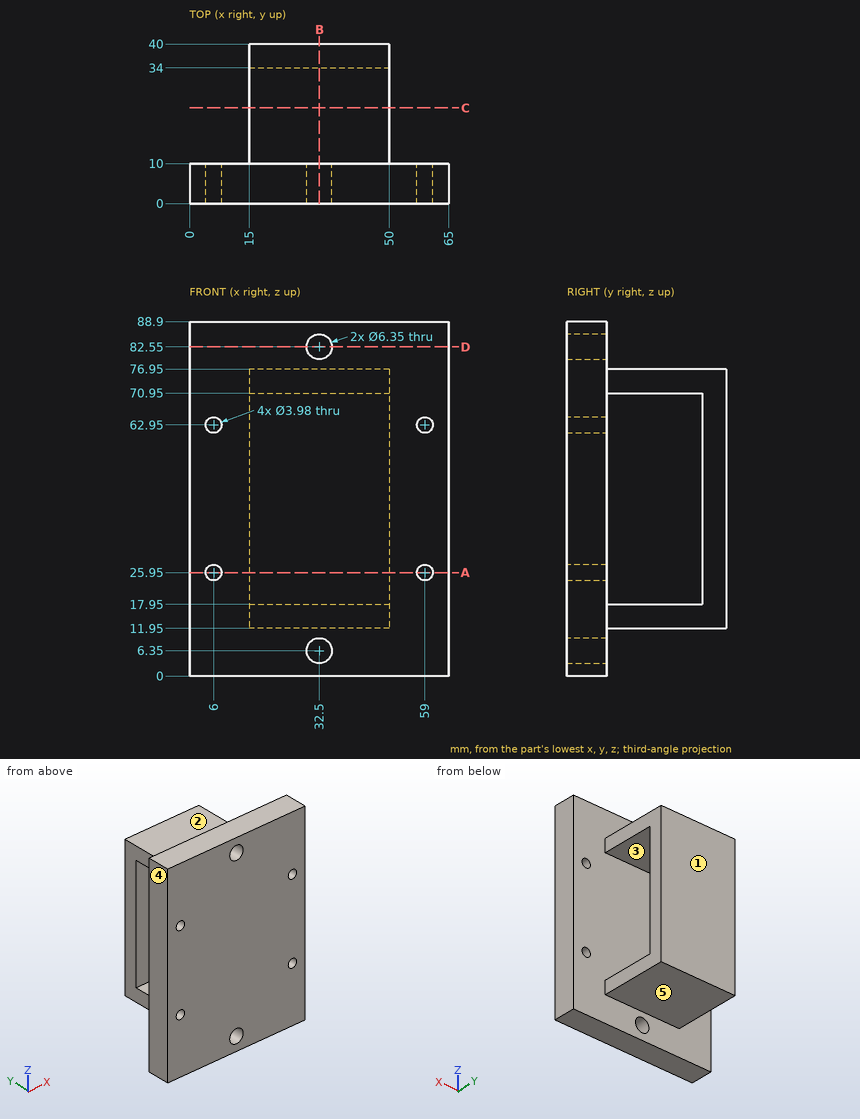
Answer from the drawing. Dimensions are ordinates in mm from the lowest x, y and z of the part. A direction names the side the tool comes from. Give positions to 0.01 mm unless a question says otherwise; leave off trailing zeros. Loops run counter-clockwise (first coordinate to the right, second up) from the corner with the lowest first, then second, coordinate; pieces in that order, holes last.
Item 1: A cutting plane is placed at D-D (z = 82.55). Give the vertices of the cut face in (x, y) (3 decimals), then the cut area to 4 significant figures.
Derived:
outline: (0, 0) - (29.325, 0) - (29.325, 10) - (0, 10) - close; (35.675, 0) - (65, 0) - (65, 10) - (35.675, 10) - close
area: 586.5 mm2
Item 2: Determine the mould class of the marked faces 1, 2 and 3 for opening direction Y: +Y half, -Y half, draft (parallel to the pull), parting line (faces both ways), or undercut.
Derived:
face 1: +Y half
face 2: draft
face 3: undercut
Item 3: A cutting plane is placed at C-C (y = 24). Give the vertices of the cut face in (x, z).
Derived:
outline: (15, 11.95) - (50, 11.95) - (50, 17.95) - (15, 17.95) - close; (15, 70.95) - (50, 70.95) - (50, 76.95) - (15, 76.95) - close
Item 4: A cutting plane is placed at A-A (z = 25.95). Give the vertices of the cut face in (x, y).
Derived:
outline: (0, 0) - (4.01, 0) - (4.01, 10) - (0, 10) - close; (7.99, 0) - (57.01, 0) - (57.01, 10) - (7.99, 10) - close; (15, 34) - (50, 34) - (50, 40) - (15, 40) - close; (60.99, 0) - (65, 0) - (65, 10) - (60.99, 10) - close
Item 5: A cutting plane is placed at B-B (x = 32.5). Give the vertices of the cut face in (y, z) (3 decimals).
Derived:
outline: (0, 0) - (10, 0) - (10, 3.175) - (0, 3.175) - close; (0, 9.525) - (10, 9.525) - (10, 11.95) - (40, 11.95) - (40, 76.95) - (10, 76.95) - (10, 79.375) - (0, 79.375) - close; (0, 85.725) - (10, 85.725) - (10, 88.9) - (0, 88.9) - close; hole (10, 17.95) - (34, 17.95) - (34, 70.95) - (10, 70.95) - close
Item 6: A tool of negligible diameter and unlimited length cuts with its end or side. For the marked faces 4 and 5, from which of +Z, -Z, +X, -X, +Y, -Y can it reach the whole face along a straight path? Write none if from no direction.
Derived:
face 4: +Z, -Z, -X, +Y, -Y
face 5: -Z, +X, -X, +Y
Item 7: Find the intervals of material crossed by line 1 along X through (y, z) = (5.25, 62.95); line 2 along Z through (x, y) = (30.5, 32.5); line 3 along Y through (x, z) = (28, 61.5), in increasing order.
Derived:
line 1: x = 0 to 4.01, 7.99 to 57.01, 60.99 to 65
line 2: z = 11.95 to 17.95, 70.95 to 76.95
line 3: y = 0 to 10, 34 to 40
Item 8: Each of these flat-tipped pins is pushed along its axis until it touches: pin 1 Ø10.5 at (x, z) = (32, 56.5) entering from -Y; pin 2 Ø3.5 at (x, z) = (59, 62.95) entering from -Y; pin 3 Ø4.5 at (x, z) = (6, 62.95) entering from +Y; pin 4 Ø3 at (x, y) = (24, 32.5) entering from -Z. Where does it stop, or does it pass through?
Derived:
pin 1: stops at y = 0
pin 2: passes through
pin 3: stops at y = 10
pin 4: stops at z = 11.95
